Verification items for the finished model (mm, model axes). A direction names the side the tool comes from. Round coordinates to 2 decimals unless told otherwise and drop trailing zeros. Order: outer loops, then holes, each group sorted by start corner. A loop starts at its lowest first (then second) coordinate and runs counter-clockwise, first axis right, second up. Notation, with made-up numbers: (80, -7.75) -> (116, -7.75) arc R24 cw to (116, 14.25) -> close; hole circle Ø10 at (59.25, 41). An arc over 180 degrees is marked (long way). Put each result on its own line as item: value.
Autodesk Inventor part; units mm, degrees
ref_plane "YZ Plane" through (0, 0, 0) normal (1, 0, 0) x (0, 1, 0)
ref_plane "XZ Plane" through (0, 0, 0) normal (0, 1, 0) x (-1, 0, 0)
ref_plane "XY Plane" through (0, 0, 0) normal (0, 0, 1) x (1, 0, 0)
sketch "Sketch1" plane through (0, 0, 0) normal (1, 0, 0) x (0, 1, 0)
  line L0 (11.1677, 16.6703) -> (5.9715, 19.6703)
  line L1 (5.9715, 19.6703) -> (0.7754, 16.6703)
  line L2 (0.7754, 16.6703) -> (0.7754, 10.6703)
  line L3 (0.7754, 10.6703) -> (5.9715, 7.6703)
  line L4 (5.9715, 7.6703) -> (11.1677, 10.6703)
  line L5 (11.1677, 10.6703) -> (11.1677, 16.6703)
  point P0 (0, 0)
  dimension "d0" = 120
  dimension "d1" = 120
  dimension "d2" = 6
extrude "Extrusion1" add sketch "Sketch1" along normal blind 5
sketch "Sketch2" plane through (5, 0, 0) normal (1, 0, 0) x (0, 0, -1)
  circle A0 centre (-13.6703, 5.9715) radius 3
  point P0 (0, 0)
  point P1 (-16.6703, 11.1677)
  point P2 (-10.6703, 0.7754)
  point P3 (-16.6703, 0.7754)
  dimension "d5" = 6
  dimension "d6" = 6
  dimension "d7" = 6
extrude "Extrusion2" add sketch "Sketch2" along normal blind 40
thread "Thread1"
chamfer "Chamfer1" distance 0.4 angle 45 1 edges at (45, 5.9715, 16.6703)
properties part number "Screw"
Item 1: Material ranges on L1, parallel to Y at x = 22, z = 13.5; L2, parallel to X at y = 1.75, z = 12.5; L3, parallel to Y at x = 23.5, z = 12.5, recorded low to high. Write a range as [from, to].
Check sheet entries:
L1: y = [2.98, 8.97]
L2: x = [0, 5]
L3: y = [3.21, 8.73]
Item 2: Tool access check on faces 1 (the flat face through (0, 6, 14)), 2 (the cylindrical face through (24.52, 7.8, 16.05)). Record the directions out of +Z, -Z, +X, -X, +Y, -Y that give a thin tool (end or side, any length) a straight path to the whole face; none if there is none.
Check sheet entries:
face 1: +Z, -Z, -X, +Y, -Y
face 2: +X
Item 3: Section check C-C on z = 9.5. Record the boundary of the cut face in (x, y).
Check sheet entries:
outline: (0, 2.8) -> (5, 2.8) -> (5, 9.14) -> (0, 9.14) -> close
Item 4: Section check A-A on x = 25. Record the boundary of the cut face in (y, z).
Check sheet entries:
outline: circle Ø6 at (5.97, 13.67)
Item 5: Section check B-B on y = 9.5. Record the boundary of the cut face in (x, z), then the cut area to 3 significant figures.
Check sheet entries:
outline: (0, 9.71) -> (5, 9.71) -> (5, 17.63) -> (0, 17.63) -> close
area: 39.6 mm^2
Item 6: Gauge pin test, flat ends, axial feed: pin 1 Ø4 at (x, z) = (33, 12.5) entering from -Y; pin 2 Ø1.5 at (x, z) = (38.5, 10.5) entering from +Y. Record the tip position at first contact, or that the pin passes through.
Check sheet entries:
pin 1: stops at y = 2.97
pin 2: stops at y = 7.74
